from build123d import *
from OCP.BRepFilletAPI import BRepFilletAPI_MakeChamfer

# Parameters (mm, degrees)
SKETCH1_W                  = 50
SKETCH1_H                  = 21
BASE_DEPTH                 = 2
SKETCH2_W                  = 50
SKETCH2_H                  = 42
SKETCH2_R                  = 2
SKETCH2_R_2                = 12.5
ENCAIXE_MOTOR_DEPTH        = 4
LATERAIS_START             = -50
LATERAIS_BLOCO_DEPTH       = 50
LATERAIS_START_2           = -17
SKETCH4_W                  = 46
SKETCH4_H                  = 40
LATERAIS_CORTE_DEPTH       = 17
SUPORTE_CENTRAL_DEPTH      = 8
SUPORTE_CENTRAL_DEPTH_BACK = 8
SKETCH6_R                  = 12.5
FURO_MOTOR_25_DEPTH        = 68.475921631
CHANFROS_1X45_SIZE         = 0.5
CHANFROS_1X45_SIZE_2       = 0.897527468
CHANFROS_2X45_SIZE         = 2


# Some blends are built 0.0001 mm under size
with BuildPart() as part:
    # Sketch1 → Base (new body)
    with BuildSketch(Plane(origin=(0, 0, 0), x_dir=(1, 0, 0), z_dir=(0, 1, 0))):
        with Locations((25, 10.5)):
            Rectangle(SKETCH1_W, SKETCH1_H)
        with BuildLine():
            Line((7.25, 11), (7.25, 10))
            ThreePointArc((7.25, 10), (5, 7.75), (2.75, 10))
            Line((2.75, 10), (2.75, 11))
            ThreePointArc((2.75, 11), (5, 13.25), (7.25, 11))
        make_face(mode=Mode.SUBTRACT)
        with BuildLine():
            Line((42.75, 11), (42.75, 10))
            ThreePointArc((42.75, 10), (45, 7.75), (47.25, 10))
            Line((47.25, 10), (47.25, 11))
            ThreePointArc((47.25, 11), (45, 13.25), (42.75, 11))
        make_face(mode=Mode.SUBTRACT)
        with BuildLine():
            Line((27.25, 16), (27.25, 15))
            ThreePointArc((27.25, 15), (25, 12.75), (22.75, 15))
            Line((22.75, 15), (22.75, 16))
            ThreePointArc((22.75, 16), (25, 18.25), (27.25, 16))
        make_face(mode=Mode.SUBTRACT)
    extrude(amount=BASE_DEPTH)

    # Sketch2 → Encaixe Motor (add)
    with BuildSketch(Plane.XY):
        with Locations((25, 21)):
            Rectangle(SKETCH2_W, SKETCH2_H)
        with Locations((9.5, 35.5)):
            Circle(SKETCH2_R, mode=Mode.SUBTRACT)
        with Locations((9.5, 4.5)):
            Circle(SKETCH2_R, mode=Mode.SUBTRACT)
        with Locations((40.5, 4.5)):
            Circle(SKETCH2_R, mode=Mode.SUBTRACT)
        with Locations((40.5, 35.5)):
            Circle(SKETCH2_R, mode=Mode.SUBTRACT)
        with Locations((25, 20)):
            Circle(SKETCH2_R_2, mode=Mode.SUBTRACT)
    extrude(amount=-ENCAIXE_MOTOR_DEPTH)

    # Sketch3 → Laterais - Bloco (add)
    with BuildSketch(Plane(origin=(50, 0, 0), x_dir=(0, 0, -1), z_dir=(1, 0, 0)).offset(LATERAIS_START)):
        with BuildLine():
            Line((21, 2), (4, 42))
            Line((4, 42), (4, 2))
            Line((4, 2), (6.5, 2))
            Line((6.5, 2), (6.5, 4))
            ThreePointArc((6.5, 4), (6.939339828, 5.060660172), (8, 5.5))
            Line((8, 5.5), (13, 5.5))
            ThreePointArc((13, 5.5), (14.060660172, 5.060660172), (14.5, 4))
            Line((14.5, 4), (14.5, 2))
            Line((14.5, 2), (21, 2))
        make_face()
    extrude(amount=LATERAIS_BLOCO_DEPTH)

    # Sketch4 → Laterais - Corte (cut)
    with BuildSketch(Plane(origin=(0, 0, -21), x_dir=(-1, 0, 0), z_dir=(0, 0, -1)).offset(LATERAIS_START_2)):
        with Locations((-25, 22)):
            Rectangle(SKETCH4_W, SKETCH4_H)
    extrude(amount=LATERAIS_CORTE_DEPTH, mode=Mode.SUBTRACT)

    # Sketch5 → Suporte Central (add, two sides: drawn at the far end of the back side and taken through both)
    with BuildSketch(Plane.ZY.offset(-25).offset(-SUPORTE_CENTRAL_DEPTH_BACK)):
        Polygon((-4, 2), (-8, 2), (-4, 12), align=None)
    extrude(amount=SUPORTE_CENTRAL_DEPTH + SUPORTE_CENTRAL_DEPTH_BACK)

    # Sketch6 → Furo Motor Ø25 (cut, through all)
    with BuildSketch(Plane.XY.offset(-4)):
        with Locations((25, 20)):
            Circle(SKETCH6_R)
    extrude(amount=-FURO_MOTOR_25_DEPTH, mode=Mode.SUBTRACT)

    # Chanfros 1x45°
    chanfros_1x45_edges_1 = [part.edges().sort_by_distance(p)[0] for p in [
        (2, 2, -17.75),
        (48, 2, -17.75),
        (48, 2, -5.25),
        (40.5, 2, -4),
        (2, 2, -5.25),
        (9.5, 2, -4),
        (33, 2, -6),
        (17, 2, -6),
    ]]
    chanfros_1x45_edges_2 = [part.edges().sort_by_distance(p)[0] for p in [
        (25, 2, -8),
    ]]
    chanfros_1x45_side_2 = [part.faces().sort_by_distance(p)[0] for p in [
        (25, 2, -8.01),
    ]]
    chanfros_1x45 = BRepFilletAPI_MakeChamfer(part.part.solid().wrapped)
    for e in chanfros_1x45_edges_1:
        chanfros_1x45.Add(CHANFROS_1X45_SIZE - 0.0001, e.wrapped)
    for e in chanfros_1x45_edges_2:
        chanfros_1x45.Add(CHANFROS_1X45_SIZE - 0.0001, CHANFROS_1X45_SIZE_2 - 0.0001, e.wrapped, chanfros_1x45_side_2[0].wrapped)
    add(Compound.cast(chanfros_1x45.Shape()), mode=Mode.REPLACE)  # a hair under: the kernel refuses the full size

    # Chanfros 2x45°
    # the kernel refuses this chamfer: 2 mm, written as the material it adds along each edge
    with BuildSketch(Plane(origin=(48, 42, -4), x_dir=(-0.9996219169112968, 0, 0.027495876610586726), z_dir=(0, -1, 0))) as chanfros_2x45_piece_1_section:
        Polygon((CHANFROS_2X45_SIZE * 0.999621916911, CHANFROS_2X45_SIZE * 0.0274958766106), (-CHANFROS_2X45_SIZE * 0.0274958766106, CHANFROS_2X45_SIZE * 0.999621916911), (0, 0), align=None)
    chanfros_2x45_piece_1 = extrude(amount=44.643465976, mode=Mode.PRIVATE)
    chanfros_2x45_piece_1 = split(chanfros_2x45_piece_1, bisect_by=Plane(origin=(47.331403888, 24.268482908, -11.535894764), z_dir=(0, -0.3911406403448519, 0.9203309184584747)), keep=Keep.TOP, mode=Mode.PRIVATE)
    chanfros_2x45_piece_1 = split(chanfros_2x45_piece_1, bisect_by=Plane(origin=(47.331403888, 11.597453936, 5.097553936), z_dir=(0, 0.7071067811865476, -0.7071067811865476)), keep=Keep.TOP, mode=Mode.PRIVATE)
    chanfros_2x45_piece_1 = split(chanfros_2x45_piece_1, bisect_by=Plane(origin=(57.08562089, 11.58552089, -4.64473002), z_dir=(-0.70710678118655, 0.707106781186545, 0)), keep=Keep.TOP, mode=Mode.PRIVATE)
    add(chanfros_2x45_piece_1)
    with BuildSketch(Plane(origin=(48, 42, -4), x_dir=(-0.9996219169112968, 0, 0.027495876610586726), z_dir=(0, -1, 0))) as chanfros_2x45_piece_2_section:
        Polygon((CHANFROS_2X45_SIZE * 0.999621916911, CHANFROS_2X45_SIZE * 0.0274958766106), (-CHANFROS_2X45_SIZE * 0.0274958766106, CHANFROS_2X45_SIZE * 0.999621916911), (0, 0), align=None)
    chanfros_2x45_piece_2 = extrude(amount=44.643465976, mode=Mode.PRIVATE)
    chanfros_2x45_piece_2 = split(chanfros_2x45_piece_2, bisect_by=Plane(origin=(47.794441496, 1.480569573, -5.019330427), z_dir=(0, 0.7071067811865476, -0.7071067811865476)), keep=Keep.TOP, mode=Mode.PRIVATE)
    chanfros_2x45_piece_2 = split(chanfros_2x45_piece_2, bisect_by=Plane(origin=(47.523184188, 2.023084188, -5.290587735), z_dir=(0.70710678118655, -0.707106781186545, 0)), keep=Keep.TOP, mode=Mode.PRIVATE)
    add(chanfros_2x45_piece_2)
    with BuildSketch(Plane(origin=(48, 42, -4), x_dir=(-0.9996219169112968, 0, 0.027495876610586726), z_dir=(0, -1, 0))) as chanfros_2x45_piece_3_section:
        Polygon((CHANFROS_2X45_SIZE * 0.999621916911, CHANFROS_2X45_SIZE * 0.0274958766106), (-CHANFROS_2X45_SIZE * 0.0274958766106, CHANFROS_2X45_SIZE * 0.999621916911), (0, 0), align=None)
    chanfros_2x45_piece_3 = extrude(amount=44.643465976, mode=Mode.PRIVATE)
    chanfros_2x45_piece_3 = split(chanfros_2x45_piece_3, bisect_by=Plane(origin=(46.709412265, 2.023084188, -4.476815812), z_dir=(0, -0.7071067811865476, 0.7071067811865476)), keep=Keep.TOP, mode=Mode.PRIVATE)
    chanfros_2x45_piece_3 = split(chanfros_2x45_piece_3, bisect_by=Plane(origin=(46.980669573, 1.480569573, -4.205558504), z_dir=(-0.70710678118655, 0.707106781186545, 0)), keep=Keep.TOP, mode=Mode.PRIVATE)
    add(chanfros_2x45_piece_3)
    with BuildSketch(Plane(origin=(2, -2.643465976, -4), x_dir=(0.9996219169112968, 0, 0.027495876610585838), z_dir=(0, 1, 0))) as chanfros_2x45_piece_4_section:
        Polygon((CHANFROS_2X45_SIZE * 0.999621916911, CHANFROS_2X45_SIZE * 0.0274958766106), (-CHANFROS_2X45_SIZE * 0.0274958766106, CHANFROS_2X45_SIZE * 0.999621916911), (0, 0), align=None)
    chanfros_2x45_piece_4 = extrude(amount=44.643465976, mode=Mode.PRIVATE)
    chanfros_2x45_piece_4 = split(chanfros_2x45_piece_4, bisect_by=Plane(origin=(2.205558504, 1.480569573, -5.019330427), z_dir=(0, 0.7071067811865476, -0.7071067811865476)), keep=Keep.TOP, mode=Mode.PRIVATE)
    chanfros_2x45_piece_4 = split(chanfros_2x45_piece_4, bisect_by=Plane(origin=(2.476815812, 2.023084188, -5.290587735), z_dir=(-0.7071067811865479, -0.7071067811865472, 0)), keep=Keep.TOP, mode=Mode.PRIVATE)
    add(chanfros_2x45_piece_4)
    with BuildSketch(Plane(origin=(2, -2.643465976, -4), x_dir=(0.9996219169112968, 0, 0.027495876610585838), z_dir=(0, 1, 0))) as chanfros_2x45_piece_5_section:
        Polygon((CHANFROS_2X45_SIZE * 0.999621916911, CHANFROS_2X45_SIZE * 0.0274958766106), (-CHANFROS_2X45_SIZE * 0.0274958766106, CHANFROS_2X45_SIZE * 0.999621916911), (0, 0), align=None)
    chanfros_2x45_piece_5 = extrude(amount=44.643465976, mode=Mode.PRIVATE)
    chanfros_2x45_piece_5 = split(chanfros_2x45_piece_5, bisect_by=Plane(origin=(3.290587735, 2.023084188, -4.476815812), z_dir=(0, -0.7071067811865476, 0.7071067811865476)), keep=Keep.TOP, mode=Mode.PRIVATE)
    chanfros_2x45_piece_5 = split(chanfros_2x45_piece_5, bisect_by=Plane(origin=(3.019330427, 1.480569573, -4.205558504), z_dir=(0.7071067811865479, 0.7071067811865472, 0)), keep=Keep.TOP, mode=Mode.PRIVATE)
    add(chanfros_2x45_piece_5)
    with BuildSketch(Plane(origin=(2, -2.643465976, -4), x_dir=(0.9996219169112968, 0, 0.027495876610585838), z_dir=(0, 1, 0))) as chanfros_2x45_piece_6_section:
        Polygon((CHANFROS_2X45_SIZE * 0.999621916911, CHANFROS_2X45_SIZE * 0.0274958766106), (-CHANFROS_2X45_SIZE * 0.0274958766106, CHANFROS_2X45_SIZE * 0.999621916911), (0, 0), align=None)
    chanfros_2x45_piece_6 = extrude(amount=44.643465976, mode=Mode.PRIVATE)
    chanfros_2x45_piece_6 = split(chanfros_2x45_piece_6, bisect_by=Plane(origin=(2.668596112, 11.597453936, 5.097553936), z_dir=(0, 0.7071067811865476, -0.7071067811865476)), keep=Keep.TOP, mode=Mode.PRIVATE)
    chanfros_2x45_piece_6 = split(chanfros_2x45_piece_6, bisect_by=Plane(origin=(-7.08562089, 11.58552089, -4.64473002), z_dir=(0.7071067811865479, 0.7071067811865472, 0)), keep=Keep.TOP, mode=Mode.PRIVATE)
    chanfros_2x45_piece_6 = split(chanfros_2x45_piece_6, bisect_by=Plane(origin=(2.668596112, 24.268482908, -11.535894764), z_dir=(0, -0.3911406403448519, 0.9203309184584747)), keep=Keep.TOP, mode=Mode.PRIVATE)
    add(chanfros_2x45_piece_6)


solid = part.part
Can you work these out from the model? Positions are in its coordinate system, mm. A direction names the side the tool comes from. Coordinates: 2 decimals unless noted, no trailing zeros. Write each loop counter-clockwise with the first axis right and the second up, starting at its lowest first coordinate (ties: lowest second). Pieces come first, ordered by that corner, then holes. Notation, with made-up numbers: (88.25, 56.5) -> (132.25, 56.5) arc R25 ccw to (132.25, 90.5) -> close; hole circle Ø6 at (-6, -10.5). An arc over 180 degrees is marked (long way). Write item = value, one per line.
(1) Imagine slicing it at B-B (x = 45). Please give me the cut outline in (y, z).
Verdict:
outline = (0, -21) -> (2, -21) -> (2, -13.25) -> (0, -13.25) -> close; (0, -7.75) -> (2, -7.75) -> (2, -4.5) -> (2.5, -4) -> (42, -4) -> (42, 0) -> (0, 0) -> close
(2) Imagine slicing it at A-A (x = 9.5). State how many separate pieces and enclosed holes the cut face has, and give its area (3 significant figures).
Verdict:
separate_pieces = 3
enclosed_holes = 0
area = 170 mm^2
(3) Imagine slicing it at C-C (y = 35.5). Please give me the cut outline in (x, z), and give its area (3 significant figures).
Verdict:
outline = (0, -6.76) -> (2, -6.76) -> (2, -6) -> (4, -4) -> (7.5, -4) -> (7.5, 0) -> (0, 0) -> close; (11.5, -4) -> (38.5, -4) -> (38.5, 0) -> (11.5, 0) -> close; (42.5, -4) -> (46, -4) -> (48, -6) -> (48, -6.76) -> (50, -6.76) -> (50, 0) -> (42.5, 0) -> close
area = 183 mm^2
(4) Imagine slicing it at D-D (y = 29). Please give me the cut outline in (x, z) (3 decimals), and give its area (3 significant figures).
Verdict:
outline = (0, -9.525) -> (2, -9.525) -> (2, -6) -> (4, -4) -> (16.325, -4) -> (16.325, 0) -> (0, 0) -> close; (33.675, -4) -> (46, -4) -> (48, -6) -> (48, -9.525) -> (50, -9.525) -> (50, 0) -> (33.675, 0) -> close
area = 157 mm^2
(5) If I drill on probe 1 along Y at (x, z) = (40.5, -2.25); probe 2 along X at (y, z) = (20, -10); probe 3 along X at (y, z) = (29, -5.5), over which ranges is the centre line in solid material (lowest first)?
Verdict:
probe_1 = 0 to 2.5, 6.5 to 33.5, 37.5 to 42
probe_2 = 0 to 2, 48 to 50
probe_3 = 0 to 2.5, 47.5 to 50
(6) On a 3-axis mill with a long thin cutter (end or side, diameter ignored), from which of +Z, -Z, +X, -X, +Y, -Y can I reach the whole of each face in a straight line? I mean faces 1 (the face through (44.95, 0.99, -7.75)), 2 (the face through (17, 6, -5)), 3 (the face through (1, 5.5, -10)), 4 (the face through (49, 3, -6.5)). Say none if no direction works.
Verdict:
face_1 = +Y, -Y
face_2 = -Z, +Y
face_3 = +X, -X
face_4 = +X
(7) Thinking about a two-plate mould opening in Y: for faces 5 (the face through (1.08, 21.72, -12.62)), 6 (the face through (0.99, 5.05, -6.93)), 7 (the face through (48, 16, -12)), which applies, +Y half, -Y half, draft (parallel to the pull), parting line (faces both ways), or undercut?
Verdict:
face_5 = +Y half
face_6 = undercut
face_7 = draft
(8) For pin 1 (12 mm diameter, centred on x = 23.5, y = 31, fed in from -Z); pin 2 (3 mm diameter, centred on x = 15.5, y = 23.5, fed in from -Z); pin 3 (0.6 mm diameter, centred on x = 49, y = 3.5, fed in from -Z); pin 4 (8.5 mm diameter, centred on x = 24.5, z = -15, fed in from +Y), each with a flat end and sliding along its axis, tell me the tip position at first contact or that it passes through.
Verdict:
pin_1 = -4
pin_2 = through
pin_3 = -20.49
pin_4 = 2
